Can you work these out from the model? Positions are in its coordinate system, mm. A direction names the side the tool comes from. Round coordinates to 2 decimals unless told otherwise and drop trailing zeros. Order: outer loops, then holes, each group sorted by start corner. A loop starts at its lowest first (then second) coordinate and runs counter-clockwise, first axis right, second up. Notation, with made-up numbers: (65, 54.5) -> (119, 54.5) arc R17 cw to (119, 82.5) -> close; hole circle Ø11 at (66, -28). An arc over 180 degrees is marked (long way). One line per item, written item: value.
```python
from build123d import *

# Parameters (mm, degrees)
F2_W     = 48.837749362
F2_H     = 47.5878509101
F2_W_2   = 45
F2_H_2   = 43.5878502545
F2_R     = 1.25
F2_R_2   = 15.75
F3_DEPTH = 5
F4_DEPTH = 50
F5_R     = 2


with BuildPart() as f3:
    # F2 (on Front) → F3 (new body)
    with BuildSketch(Plane.XZ):
        with Locations((0.0811256468, 0)):
            Rectangle(F2_W, F2_H)
        Rectangle(F2_W_2, F2_H_2, mode=Mode.SUBTRACT)
        Rectangle(F2_W_2, F2_H_2)
        with Locations((-17.6653114055, -17.6373357058)):
            Circle(F2_R, mode=Mode.SUBTRACT)
        Circle(F2_R_2, mode=Mode.SUBTRACT)
        with Locations((17.6900276539, 17.7180033535)):
            Circle(F2_R, mode=Mode.SUBTRACT)
    extrude(amount=F3_DEPTH)

    # F2 (on Front) → F4 (join)
    with BuildSketch(Plane.XZ):
        with Locations((0.0811256468, 0)):
            Rectangle(F2_W, F2_H)
        Rectangle(F2_W_2, F2_H_2, mode=Mode.SUBTRACT)
    extrude(amount=F4_DEPTH)

    # F5
    f5_edges = [f3.edges().sort_by_distance(p)[0] for p in [
        (-24.337749, -25, 23.793925),
        (24.5, -25, 23.793925),
        (24.5, -25, -23.793925),
        (-24.337749, -25, -23.793925),
    ]]
    fillet(f5_edges, radius=F5_R)


solid = f3.part
```
Q1. I want a section at A-A on x = 0. List the corners of the cut face in (y, z) for me.
Answers below:
outline: (-50, -23.79) -> (0, -23.79) -> (0, -15.75) -> (-5, -15.75) -> (-5, -21.79) -> (-50, -21.79) -> close; (-50, 21.79) -> (-5, 21.79) -> (-5, 15.75) -> (0, 15.75) -> (0, 23.79) -> (-50, 23.79) -> close
Q2. Please list where these lines run through material, in increasing order: line 1 along Z through (x, y) = (-3, -17.5); line 2 along X through (y, z) = (-16, -10.5); line 3 along Z through (x, y) = (0, -2.85).
Answers below:
line 1: -23.79 to -21.79, 21.79 to 23.79
line 2: -24.34 to -22.5, 22.5 to 24.5
line 3: -23.79 to -15.75, 15.75 to 23.79
Q3. Will this pin go through, and if not, where does the flat tip stop? pin 1 Ø3 at (x, z) = (17.69, 17.72) entering from -Y.
Answers below:
pin 1: y = -5
Q4. I want a section at D-D on x = 21.5. List the corners of the cut face in (y, z) for me.
Answers below:
outline: (-50, -23.79) -> (0, -23.79) -> (0, 23.79) -> (-50, 23.79) -> (-50, 21.79) -> (-5, 21.79) -> (-5, -21.79) -> (-50, -21.79) -> close
Q5. I want a section at B-B on z = 0. List the corners of the cut face in (x, y) for me.
Answers below:
outline: (-24.34, -50) -> (-22.5, -50) -> (-22.5, -5) -> (-15.75, -5) -> (-15.75, 0) -> (-24.34, 0) -> close; (15.75, -5) -> (22.5, -5) -> (22.5, -50) -> (24.5, -50) -> (24.5, 0) -> (15.75, 0) -> close
Q6. On a 3-axis mill with a long thin cutter (end or side, diameter ignored), from which of +Z, -Z, +X, -X, +Y, -Y can I reach the whole of each face in a straight line? I mean faces 1 (the face through (-22.5, -27, 0)), 2 (the face through (-24.338, -25, 0)). Say none if no direction works.
Answers below:
face 1: -Y
face 2: +Z, -Z, -X, +Y, -Y
Q7. I want a section at C-C on y = -41.5. List the corners of the cut face in (x, z) for me.
Answers below:
outline: (-24.34, -21.79) arc R2 ccw to (-22.34, -23.79) -> (22.5, -23.79) arc R2 ccw to (24.5, -21.79) -> (24.5, 21.79) arc R2 ccw to (22.5, 23.79) -> (-22.34, 23.79) arc R2 ccw to (-24.34, 21.79) -> close; hole (-22.5, -21.79) -> (22.5, -21.79) -> (22.5, 21.79) -> (-22.5, 21.79) -> close
Q8. We'd pull the mould along X, two halves only. Please class faces 3 (the face through (0, -25, -23.794)), 4 (the face through (-23.77, -25.35, -23.19)), 5 (the face through (-17.936, -2.465, -18.858)): released by +X, released by -X, zero draft, split by the parting line, or undercut.
Answers below:
face 3: zero draft
face 4: released by -X
face 5: undercut
